Design review of the part built by this model. Coordinates are the model's own, in mm. A direction names the side the tool comes from. Coordinates: 2 decimals unless noted, no trailing zeros. Loops run counter-clockwise (first coordinate to the right, second up) from the corner with the lowest first, then second, coordinate; pieces in that order, holes last. Notation, with made-up numbers: (-37.5, 24) -> (0.5, 24) arc R20 cw to (0.5, 60) -> close; hole circle Ø8 at (51.5, 64). An arc over 180 degrees is marked (long way). Use one line per item in the form item = value. Start each with the question number.
1. Machinability: for faces 1 (the face through (20, -250, 483)), 2 (the face through (255, -3, 281)), 3 (the face through (765, -148.4, 772)), which of the approach directions +Z, -Z, +X, -X, +Y, -Y give a long, thin tool a straight path to every point of the face, cutting with its end or side? Answer none if there is none.
2. Consider section B-B (z = 589). State the section outline as (x, y) points.
3. For pin 1 (1 mm diameter, centred on y = -27.5, z = 557, fed in from +X); pin 2 (1.5 mm diameter, centred on x = 52.5, y = 128, fed in from -Z); pin 3 (5 mm diameter, centred on x = 419, y = 35.5, fed in from -Z), all flat-tipped, find the tip position at first contact; note any pin that passes through.
4. Consider section A-A (y = -218). State the section outline as (x, z) points, then the cut area to 3 significant figures.
5. Consider section D-D (x = 642). State the section outline as (y, z) points.
6. Wall thickness on line 1 (Y direction, x = 728, z = 719); line 2 (Z direction, x = 477, y = 43); line 3 (X direction, y = -18, z = 130.5): over which ranges is each line inside the solid? List them lowest first. Write a range as from..to.
7. Consider section C-C (x = 297). State the section outline as (y, z) points, then the cut area to 4 significant figures.
from build123d import *

# Parameters (mm, degrees)
SKIZZE7_W                       = 510
SKIZZE7_H                       = 500
AUFSATZ_LINEAR_AUSTRAGEN1_DEPTH = 979
SKIZZE8_W                       = 409
SKIZZE8_H                       = 398.4
AUFSATZ_LINEAR_AUSTRAGEN2_DEPTH = 1222.75
SKIZZE9_W                       = 409
SKIZZE9_H                       = 500
AUFSATZ_LINEAR_AUSTRAGEN3_DEPTH = 721.15
FORMSCHR_GE1_ANGLE              = 45


with BuildPart() as part:
    # Skizze7 → Aufsatz-Linear austragen1 (new body)
    with BuildSketch(Plane.XY):
        Rectangle(SKIZZE7_W, SKIZZE7_H)
    extrude(amount=AUFSATZ_LINEAR_AUSTRAGEN1_DEPTH)

    # Skizze8 → Aufsatz-Linear austragen2 (add)
    with BuildSketch(Plane.ZY.offset(255)):
        with Locations((774.5, 50.8)):
            Rectangle(SKIZZE8_W, SKIZZE8_H)
    extrude(amount=-AUFSATZ_LINEAR_AUSTRAGEN2_DEPTH)

    # Skizze9 → Aufsatz-Linear austragen3 (add)
    with BuildSketch(Plane.ZY.offset(255)):
        with Locations((774.5, 0)):
            Rectangle(SKIZZE9_W, SKIZZE9_H)
    extrude(amount=-AUFSATZ_LINEAR_AUSTRAGEN3_DEPTH)

    # Formschräge1
    formschr_ge1_faces = [part.faces().sort_by_distance(p)[0] for p in [
        (466.15, -199.2, 774.5),
    ]]
    draft(formschr_ge1_faces, Plane(origin=(-255, -250, 979), x_dir=(0, 0, -1), z_dir=(0, -1, 0)), FORMSCHR_GE1_ANGLE)


solid = part.part
Geometry check:
q1.face_1 = +Z, -Z, +X, -X, -Y
q1.face_2 = -Z, +X, +Y, -Y
q1.face_3 = +Z, -Z, +X, -Y
q2.outline = (-255, -250) -> (466.15, -250) -> (567.75, -148.4) -> (967.75, -148.4) -> (967.75, 250) -> (-255, 250) -> close
q3.pin_1 = 255
q3.pin_2 = 0
q3.pin_3 = 570
q4.outline = (-255, 0) -> (255, 0) -> (255, 570) -> (498.15, 570) -> (498.15, 979) -> (-255, 979) -> close
q4.area = 599,000 mm²
q5.outline = (-148.4, 570) -> (250, 570) -> (250, 979) -> (-148.4, 979) -> close
q6.line_1 = -148.4..250
q6.line_2 = 570..979
q6.line_3 = -255..255
q7.outline = (-250, 570) -> (250, 570) -> (250, 979) -> (-250, 979) -> close
q7.area = 204,500 mm²
